Source: CAD feature listing. Evaluate the final solid. Frame: model axes, mm. Face numbers are marked on the shaded views. A direction names the side the tool comes from. Round coordinates to 2 decimals unless told otherwise and drop trailing zeros. Order: outer loops, then holes, each group sorted by start corner. A loop starts at its lowest first (then second) coordinate and runs counter-clockwise, first axis right, second up. Notation, with made-up numbers: M -36,20.25 L 11,20.25 A18 ccw 11,24.25 Z; hole C 13,43 d7. An arc over 180 degrees is marked long. Use one line per item in the form item = value. Start each with the question number.
Q1. Reachability of the marked faces 5, 6 and 7 from +Z, -Z, +X, -X, +Y, -Y: full face, straight path, thin tool, end or side. Return the list, or none.
Q2. Pull-direction query (Z, two-part tool) for the marked faces 1, 2, 3 and 4; classes: pulls with the +Z half, pulls with the -Z half, needs draft (parallel to the pull), parting line crosses it, or undercut.
Q3. Section B-B (z = 41.5). Return the cut outline in (x, y), plus the area to 3 significant figures.
Q4. Material intervals for probe 1 along Z at (x, y) = (28, 14.5); probe 2 along Z at (x, y) = (-11.5, 8); probe 3 along Z at (x, y) = (2, 53), sorted ascending.
Q5. Section C-C (y = 51). Return the cut outline in (x, z), plus the area to 3 significant figures.
Q6. Section A-A (z = 51). Give the number of separate pieces and of enclosed holes in the cut face, plus the area to 3 significant figures.
Q7. Contact query for flat-ended pins moving along their axis: pin 1 (12 mm diameter, centred on x = -7.5, z = 20, fed in from +Y); pin 2 (0.6 mm diameter, centred on x = 47.5, z = 51, fed in from -Y); pin 3 (1.4 mm diameter, centred on x = -10, z = 50, fed in from +Y). Output: stop coordinate, or through.
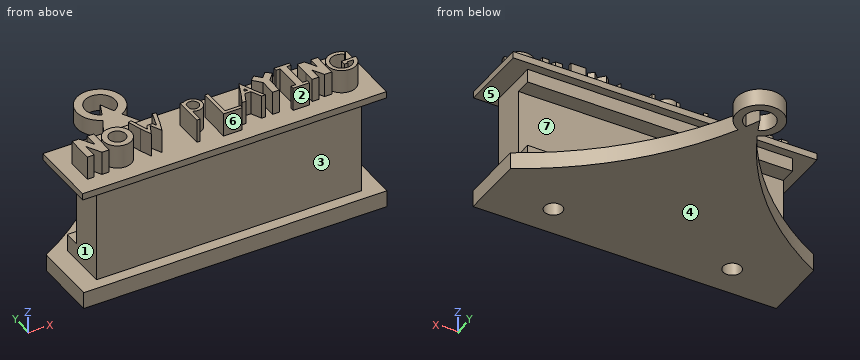
from build123d import *

# Parameters (mm, degrees)
F1_DEPTH  = 6.35
F3_DEPTH  = 6.35
F5_DEPTH  = 25.4
F7_D      = 6.7564
F7_DEPTH  = 12.7
F7_TIP    = 2.0298273432
F9_DEPTH  = 5.08
F10_W     = 99.64261204
F10_H     = 18.998793792
F11_DEPTH = 2.54
F12_R     = 5.2534292615
F12_R_2   = 3.1134110093
F13_DEPTH = 8.89


with BuildPart() as f1:
    # F0 (on Top) → F1 (new body)
    with BuildSketch(Plane.XY):
        with BuildLine():
            Line((-56.9999665022, -11.8391886353), (0, -11.8391886353))
            Line((0, -11.8391886353), (56.9999665022, -11.8391886353))
            Line((56.9999665022, -11.8391886353), (56.9999665022, 12.603007257))
            ThreePointArc((56.9999665022, 12.603007257), (25.9733436303, 36.3780469183), (3.5801271207, 68.4162692798))
            ThreePointArc((3.5801271207, 68.4162692798), (0, 85.1150162439), (-3.5801271207, 68.4162692798))
            ThreePointArc((-3.5801271207, 68.4162692798), (-25.9733436303, 36.3780469183), (-56.9999665022, 12.603007257))
            Line((-56.9999665022, 12.603007257), (-56.9999665022, -11.8391886353))
        make_face()
        with BuildLine():
            ThreePointArc((2.2622125896, 71.1828075513), (1.1022822123, 73.769792923), (0, 76.3818621635))
            ThreePointArc((0, 76.3818621635), (-1.1022822123, 73.769792923), (-2.2622125896, 71.1828075513))
            ThreePointArc((-2.2622125896, 71.1828075513), (0, 82.0517629264), (2.2622125896, 71.1828075513))
        make_face(mode=Mode.SUBTRACT)
    extrude(amount=F1_DEPTH)

    # F2 (on face) → F3 (join)
    with BuildSketch(Plane.XY.offset(6.35)):
        Polygon((0, -7.67345028), (0, 0), (0, 11.325343512), (-49.82130602, 11.325343512), (-49.82130602, -7.67345028), align=None)
        Polygon((0, 11.325343512), (0, 0), (0, -7.67345028), (49.82130602, -7.67345028), (49.82130602, 11.325343512), align=None)
    extrude(amount=F3_DEPTH)

    # F4 (on face) → F5 (join)
    with BuildSketch(Plane.XY.offset(12.7)):
        Polygon((0, -7.67345028), (0, 0), (0, 5.2618985064), (-49.82130602, 5.2618985064), (-49.82130602, -7.67345028), align=None)
        Polygon((0, 5.2618985064), (0, 0), (0, -7.67345028), (49.82130602, -7.67345028), (49.82130602, 5.2618985064), align=None)
    extrude(amount=F5_DEPTH)

    # F7
    with Locations(Plane(origin=(0, 0, 0), x_dir=(1, 0, 0), z_dir=(0, 0, -1))):
        with Locations((33.5948169231, 0), (-33.5948169231, 0)):
            Hole(F7_D / 2, depth=F7_DEPTH)
            with Locations((0, 0, -(F7_DEPTH + F7_TIP / 2))):  # 118° drill point
                Cone(0, F7_D / 2, F7_TIP, mode=Mode.SUBTRACT)

    # F8 (on face) → F9 (join)
    with BuildSketch(Plane.XY.offset(38.1)):
        Polygon((49.82130602, 11.325343512), (0, 11.325343512), (-49.82130602, 11.325343512), (-49.82130602, 5.2618985064), (49.82130602, 5.2618985064), align=None)
        Polygon((49.82130602, 5.2618985064), (-49.82130602, 5.2618985064), (-49.82130602, -7.67345028), (0, -7.67345028), (49.82130602, -7.67345028), align=None)
    extrude(amount=F9_DEPTH)

    # F10 (on face) → F11 (join)
    with BuildSketch(Plane.XY.offset(43.18)):
        Polygon((57.0974387228, 14.5591804758), (0, 14.5591804758), (-57.0974387228, 14.5591804758), (-57.0974387228, -11.3115180284), (0, -11.3115180284), (57.0974387228, -11.3115180284), align=None)
        with Locations((0, 1.825946616)):
            Rectangle(F10_W, F10_H, mode=Mode.SUBTRACT)
        with Locations((0, 1.825946616)):
            Rectangle(F10_W, F10_H)
    extrude(amount=F11_DEPTH)

    # F12 (on face) → F13 (join)
    with BuildSketch(Plane.XY.offset(45.72)):
        Polygon((8.5808153566, -3.8332685363), (10.3769853802, 0), (11.520545464, 0), (12.6641055479, 0), (14.4602755714, -3.8332685363), (15.8660151064, -3.8332685363), (14.0469819307, 0), (11.520545464, 5.8634341694), (8.9941089973, 0), (7.1750758216, -3.8332685363), align=None)
        Polygon((12.1168879583, 1.27), (10.9242029697, 1.27), (11.520545464, 2.6540106426), align=None, mode=Mode.SUBTRACT)
        Polygon((15.9370799004, 5.4188976225), (18.6398400772, 2.4412850335), (18.6398400772, -3.8332685363), (21.1798400772, -3.8332685363), (21.1798400772, 2.4412850335), (23.8826002539, 5.4188976225), (22.0018450558, 7.1260472599), (19.9098400772, 4.821299538), (17.8178350986, 7.1260472599), align=None)
        with Locations((-37.5246331096, 0)):
            Circle(F12_R)
        with Locations((-37.5246331096, 0)):
            Circle(F12_R_2, mode=Mode.SUBTRACT)
        Polygon((-49.1576491702, -5.0597838126), (-49.1576491702, 0), (-49.1576491702, 0.1703951603), (-46.2440352845, -5.0597838126), (-46.0602679443, -5.0597838126), (-43.5202679443, -5.0597838126), (-43.5202679443, 0), (-43.5202679443, 5.0597838126), (-46.0602679443, 5.0597838126), (-46.0602679443, 0), (-46.0602679443, -0.1703951603), (-48.0481869093, 3.398084528), (-49.1576491702, 5.0597838126), (-51.6976491702, 5.0597838126), (-51.6976491702, 0), (-51.6976491702, -5.0597838126), align=None)
        Polygon((-30.4608233273, 5.0550824963), (-28.8462378085, 0), (-27.2316522896, -4.2287833057), (-25.2138245851, 0), (-23.1959968805, -4.2287833057), (-21.5814113617, 0), (-19.9668258429, 5.0550824963), (-21.2886028552, 5.4772560265), (-23.3462245652, -0.964922086), (-24.0676257065, 0.5469260742), (-26.0552410036, 0.5746004754), (-26.9999829904, -1.2750737017), (-27.6364480741, 0.3864049672), (-27.6471869469, 0.4200271491), (-29.2510335929, 5.4414874634), align=None)
        with BuildLine():
            Line((-9.2688109726, -4.9615180284), (-9.2688109726, 0))
            ThreePointArc((-9.2688109726, 0), (-3.9849187402, 2.9317170847), (-9.2688109726, 5.8634341694))
            Line((-9.2688109726, 5.8634341694), (-10.5388109726, 5.8634341694))
            Line((-10.5388109726, 5.8634341694), (-10.5388109726, -4.9615180284))
            Line((-10.5388109726, -4.9615180284), (-9.2688109726, -4.9615180284))
        make_face()
        with BuildLine():
            ThreePointArc((-9.2688109726, 4.1773487671), (-5.2276091663, 2.9317170847), (-9.2688109726, 1.6860854024))
            Line((-9.2688109726, 1.6860854024), (-9.2688109726, 4.1773487671))
        make_face(mode=Mode.SUBTRACT)
        Polygon((0, -5.0356499851), (0, 0), (0, 5.8682430536), (-1.27, 5.8682430536), (-1.27, -5.0356499851), (-1.27, -6.3056499851), (0, -6.3056499851), (5.7602738962, -6.3056499851), (5.7602738962, -5.0356499851), (1.27, -5.0356499851), align=None)
        Polygon((27.2789596426, 6.2596681528), (27.2789596426, -3.9345640689), (25.489365682, -3.9345640689), (25.489365682, -5.2045640689), (28.5489596426, -5.2045640689), (31.6085536033, -5.2045640689), (31.6085536033, -3.9345640689), (29.8189596426, -3.9345640689), (29.8189596426, 6.2596681528), (31.4045827836, 6.2596681528), (31.4045827836, 7.5296681528), (28.5489596426, 7.5296681528), (25.6933365017, 7.5296681528), (25.6933365017, 6.2596681528), align=None)
        Polygon((35.9326937389, -4.0353834629), (35.9326937389, 0), (35.9283116314, 0.4862386956), (36.5847326672, -0.6176642146), (38.2620843736, -3.6311536096), (38.4455657411, -3.6311536096), (40.9855657411, -3.6311536096), (40.9855657411, 5.6661283597), (38.4455657411, 5.6661283597), (38.4455657411, 1.2884770307), (36.0522442713, 5.638557907), (35.8818776127, 5.638557907), (33.3418776127, 5.638557907), (33.3926937389, 0), (33.3926937389, -4.0353834629), align=None)
        with BuildLine():
            Line((50.4276491702, 0), (46.7712655663, 0))
            Line((46.7712655663, 0), (46.7712655663, -1.8991101533))
            Line((46.7712655663, -1.8991101533), (48.0412655663, -1.8991101533))
            Line((48.0412655663, -1.8991101533), (48.0412655663, -1.27))
            Line((48.0412655663, -1.27), (50.4594443439, -1.27))
            ThreePointArc((50.4594443439, -1.27), (42.9814431355, -0.9234763875), (49.461772222, 2.8243117093))
            Line((49.461772222, 2.8243117093), (50.4276491702, 3.852418304))
            ThreePointArc((50.4276491702, 3.852418304), (41.6742187173, -1.493446104), (51.9285291671, -1.27))
            ThreePointArc((51.9285291671, -1.27), (52.043941209, -0.6396557001), (52.0825994711, 0))
            Line((52.0825994711, 0), (50.4276491702, 0))
        make_face()
    extrude(amount=F13_DEPTH)


solid = f1.part
Results list:
q1.face_5 = none
q1.face_6 = +Z, +X, -X, -Y
q1.face_7 = +X, -X, +Y
q2.face_1 = undercut
q2.face_2 = needs draft
q2.face_3 = undercut
q2.face_4 = pulls with the -Z half
q3.outline = M -49.82,-7.67 L 49.82,-7.67 L 49.82,11.33 L -49.82,11.33 Z
q3.area = 1,890 mm2
q4.probe_1 = 0 to 6.35, 43.18 to 45.72
q4.probe_2 = 0 to 12.7, 38.1 to 45.72
q4.probe_3 = 0 to 6.35
q5.outline = M -13.92,0 L 13.92,0 L 13.92,6.35 L -13.92,6.35 Z
q5.area = 177 mm2
q6.separate_pieces = 10
q6.enclosed_holes = 3
q6.area = 412 mm2
q7.pin_1 = 5.26
q7.pin_2 = -5.29
q7.pin_3 = 5.86
